Work out the finished part from the listing and answer in its coordinate system (mm). Give positions to 0.01 mm unless a question says otherwise; leave off trailing zeros. Write each loop counter-clockwise with the first axis right and the second up, starting at its lowest first coordinate (ties: lowest second). Pieces come first, ordered by that corner, then holes. Notation, with made-up numbers: (58, -19) -> (83, -19) arc R22 cw to (83, 13) -> close; hole circle Ø1 at (70, 54.25). An arc over 180 degrees is marked (long way). Write item = value, one per line. Start each with the question number.
from build123d import *

# Parameters (mm, degrees)
F0_W     = 15.24
F0_H     = 15.24
F0_R     = 3.81
F0_W_2   = 50.8
F0_H_2   = 50.8
F1_DEPTH = 1.5875


# Not quite as in the source:
# - a feature names something its author has since deleted; it is built from what else it names


with BuildPart() as f1:
    # F0 (on Top) → F1 (new body)
    with BuildSketch(Plane.XY):
        with Locations((-39.3306643713, -48.6370485475)):
            Rectangle(F0_W, F0_H)
        with Locations((-39.3306643713, -48.6370485475)):
            Circle(F0_R, mode=Mode.SUBTRACT)
        with Locations((26.7093356287, -48.6370485475)):
            Rectangle(F0_W, F0_H)
        with Locations((26.7093356287, -48.6370485475)):
            Circle(F0_R, mode=Mode.SUBTRACT)
        with Locations((-39.3306643713, 17.4029514525)):
            Rectangle(F0_W, F0_H)
        with Locations((-39.3306643713, 17.4029514525)):
            Circle(F0_R, mode=Mode.SUBTRACT)
        with Locations((26.7093356287, 17.4029514525)):
            Rectangle(F0_W, F0_H)
        with Locations((26.7093356287, 17.4029514525)):
            Circle(F0_R, mode=Mode.SUBTRACT)
        with Locations((-6.3106643713, 17.4029514525)):
            Rectangle(F0_W_2, F0_H)
        with Locations((-6.3106643713, -48.6370485475)):
            Rectangle(F0_W_2, F0_H)
        with Locations((-39.3306643713, -15.6170485475)):
            Rectangle(F0_W, F0_H_2)
        with Locations((26.7093356287, -15.6170485475)):
            Rectangle(F0_W, F0_H_2)
    extrude(amount=F1_DEPTH)


solid = f1.part
(1) A cutting plane is placed at D-D, the plane z = 0.25. Write down the section's boundary in (x, y), then the cut area to 3 significant figures.
(2) A cutting plane is placed at C-C, the plane x = 24. Write down the section's boundary in (y, z).
(3) This flat-tipped pin is pushed along its axis until it touches: pin 1 (6 mm diameter, centred on x = -39.33, y = 17.4, fed in from -Z). Where does it stop, or does it pass through?
(4) Find the intervals of material crossed by line 1 along X through (y, z) = (-33.5, 0.45); line 2 along Y through (x, z) = (9, 0.4); line 3 along Y through (x, z) = (26.5, 1.45), in increasing order.
(5) A cutting plane is placed at B-B, the plane y = 0. Write down the section's boundary in (x, z).
(6) Determine the mould class of faces 1 (the flat face through (-7, 12, 1.588)), 2 (the cylindrical face through (28.758, -45.424, 0.783)) for opening direction Y: pulls with the +Y half, pulls with the -Y half, needs draft (parallel to the pull), parting line crosses it, or undercut.
(7) A cutting plane is placed at A-A, the plane x = -22.5. Write down the section's boundary in (y, z), then the cut area to 3 significant figures.
Results list:
q1.outline = (-46.95, -56.26) -> (34.33, -56.26) -> (34.33, 25.02) -> (-46.95, 25.02) -> close; hole circle Ø7.62 at (-39.33, -48.64); hole circle Ø7.62 at (-39.33, 17.4); hole (-31.71, -41.02) -> (19.09, -41.02) -> (19.09, 9.78) -> (-31.71, 9.78) -> close; hole circle Ø7.62 at (26.71, -48.64); hole circle Ø7.62 at (26.71, 17.4)
q1.area = 3,840 mm²
q2.outline = (-56.26, 0) -> (-51.32, 0) -> (-51.32, 1.59) -> (-56.26, 1.59) -> close; (-45.96, 0) -> (14.72, 0) -> (14.72, 1.59) -> (-45.96, 1.59) -> close; (20.08, 0) -> (25.02, 0) -> (25.02, 1.59) -> (20.08, 1.59) -> close
q3.pin_1 = through
q4.line_1 = -46.95 to -31.71, 19.09 to 34.33
q4.line_2 = -56.26 to -41.02, 9.78 to 25.02
q4.line_3 = -56.26 to -52.44, -44.83 to 13.6, 21.21 to 25.02
q5.outline = (-46.95, 0) -> (-31.71, 0) -> (-31.71, 1.59) -> (-46.95, 1.59) -> close; (19.09, 0) -> (34.33, 0) -> (34.33, 1.59) -> (19.09, 1.59) -> close
q6.face_1 = needs draft
q6.face_2 = undercut
q7.outline = (-56.26, 0) -> (-41.02, 0) -> (-41.02, 1.59) -> (-56.26, 1.59) -> close; (9.78, 0) -> (25.02, 0) -> (25.02, 1.59) -> (9.78, 1.59) -> close
q7.area = 48.4 mm²
